```python
from build123d import *

# Parameters (mm, degrees)
SKETCH1_R           = 4
BOSS_EXTRUDE1_DEPTH = 18.5
SKETCH2_W           = 25
SKETCH2_H           = 26.496950103
CUT_EXTRUDE1_DEPTH  = 50


with BuildPart() as part:
    # Sketch1 → Boss-Extrude1 (new body, symmetric)
    with BuildSketch(Plane.XY):
        with BuildLine():
            Line((-41.034119288, 1.698977617), (-44.137554517, -20))
            Line((-44.137554517, -20), (44.137554517, -20))
            Line((44.137554517, -20), (41.034119288, 1.698977617))
            ThreePointArc((41.034119288, 1.698977617), (29.475850132, 11.995709866), (17.38368573, 2.331557498))
            Line((17.38368573, 2.331557498), (17.208208741, 1.445628335))
            ThreePointArc((17.208208741, 1.445628335), (14.438314301, -3.182029332), (9.360665895, -5))
            Line((9.360665895, -5), (-9.360665895, -5))
            ThreePointArc((-9.360665895, -5), (-14.438314301, -3.182029332), (-17.208208741, 1.445628335))
            Line((-17.208208741, 1.445628335), (-17.38368573, 2.331557498))
            ThreePointArc((-17.38368573, 2.331557498), (-29.475850132, 11.995709866), (-41.034119288, 1.698977617))
        make_face()
        with Locations((29.155, 0)):
            Circle(SKETCH1_R, mode=Mode.SUBTRACT)
        with Locations((-29.155, 0)):
            Circle(SKETCH1_R, mode=Mode.SUBTRACT)
    extrude(amount=BOSS_EXTRUDE1_DEPTH, both=True)

    # Sketch2 → Cut-Extrude1 (cut, symmetric)
    with BuildSketch(Plane(origin=(0, 0, 0), x_dir=(0, 0, -1), z_dir=(1, 0, 0))):
        with Locations((0, 1.248475052)):
            Rectangle(SKETCH2_W, SKETCH2_H)
    extrude(amount=CUT_EXTRUDE1_DEPTH, both=True, mode=Mode.SUBTRACT)


solid = part.part
```
Work out the finished part from the listing and answer in its coordinate system (mm). A direction names the side the tool comes from. Give positions to 0.01 mm unless a question says otherwise; leave off trailing zeros. Order: outer loops, then holes, each group sorted by start corner. A loop starts at its lowest first (then second) coordinate and runs counter-clockwise, first axis right, second up. Notation, with made-up numbers: (84, 23) - (130, 23) arc R27 cw to (130, 58) - close; hole circle Ø1 at (75.25, 60). An arc over 180 degrees is marked (long way). One line per item, written item: value. Start each with the question number.
1. For a pull along Z with two mould halves and no side action, classify faces 1 (the face through (1, -6, -12.5)), 2 (the face through (-32.33, -2.43, -15.54)) as released by +Z, released by -Z, zero draft, split by the parting line, or undercut.
2. Section B-B, the plane y = 6.5 is taken. Write down the section's boundary in (x, z).
3. Consider line 1 (Z direction, x = -36, y = -5); line 2 (X direction, y = 0, z = -16) (3 decimals); line 3 (Y direction, x = -39, z = 4.5). Determine where each line is inside the solid, lowest interval first.
4. Section A-A, the plane z = 14 is taken. Write down the section's boundary in (x, y) (3 decimals), then the cut area to 3 significant figures.
5. Section D-D, the plane y = 0 is taken. Count the separate pieces of the cut face and the enclosed holes in it, then the cut area to 3 significant figures.
6. Each of these flat-tipped pins is pushed along its axis until it touches: pin 1 Ø5 at (x, z) = (-2, 16) entering from +Y; pin 2 Ø9 at (x, y) = (29.155, 0) entering from +Z; pin 3 Ø5 at (y, z) = (-16, 8) entering from +X; pin 4 Ø5 at (x, z) = (-25, 5) entering from +Y. Where does it stop, or does it pass through?
7. Section C-C, the plane x = 27 is taken. Write down the section's boundary in (y, z), then the cut area to 3 significant figures.
8. Which of the six approach directions +Z, -Z, +X, -X, +Y, -Y give full straight-line access (tool end or side, diameter ignored) to faces 3 (the face through (1, -12, 0)), 4 (the face through (43.297, -14.124, 0.259)), 5 (the face through (-14.38, -3.23, -15.46))?
Filled sheet:
1. face 1: undercut
1. face 2: zero draft
2. outline: (-39.24, -18.5) - (-19.07, -18.5) - (-19.07, -12.5) - (-39.24, -12.5) - close; (-39.24, 12.5) - (-19.07, 12.5) - (-19.07, 18.5) - (-39.24, 18.5) - close; (19.07, -18.5) - (39.24, -18.5) - (39.24, -12.5) - (19.07, -12.5) - close; (19.07, 12.5) - (39.24, 12.5) - (39.24, 18.5) - (19.07, 18.5) - close
3. line 1: -18.5 to -12.5, 12.5 to 18.5
3. line 2: -41.277 to -33.155, -25.155 to -16.777, 16.777 to 25.155, 33.155 to 41.277
3. line 3: -20 to -12
4. outline: (-44.138, -20) - (44.138, -20) - (41.034, 1.699) arc R12 ccw to (17.384, 2.332) - (17.208, 1.446) arc R8 cw to (9.361, -5) - (-9.361, -5) arc R8 cw to (-17.208, 1.446) - (-17.384, 2.332) arc R12 ccw to (-41.034, 1.699) - close; hole circle Ø8 at (-29.155, 0); hole circle Ø8 at (29.155, 0)
4. area: 1,910 mm²
5. separate pieces: 8
5. enclosed holes: 0
5. area: 396 mm²
6. pin 1: y = -5
6. pin 2: z = 18.5
6. pin 3: x = 43.92
6. pin 4: y = -12
7. outline: (-20, -18.5) - (-3.37, -18.5) - (-3.37, -12.5) - (-12, -12.5) - (-12, 12.5) - (-3.37, 12.5) - (-3.37, 18.5) - (-20, 18.5) - close; (3.37, -18.5) - (11.8, -18.5) - (11.8, -12.5) - (3.37, -12.5) - close; (3.37, 12.5) - (11.8, 12.5) - (11.8, 18.5) - (3.37, 18.5) - close
7. area: 501 mm²
8. face 3: +X, -X, +Y
8. face 4: +Z, -Z, +X, +Y
8. face 5: +Z, -Z, +Y
